```python
from build123d import *

# Parameters (mm, degrees)
F0_R     = 11
F1_DEPTH = 14.1
F2_R     = 11.385
F3_DEPTH = 28.4
F5_DEPTH = 17.5
F7_R     = 0.4828427125


# Not quite as in the source:
# - a fillet or chamfer that OpenCascade refuses, or shapes differently, is made with other operations: its cross-section is extruded or revolved along the edge and cut away or added


with BuildPart() as f1:
    # F0 (on Top) → F1 (new body)
    with BuildSketch(Plane.XY):
        with Locations((0, -12.3603016903)):
            Circle(F0_R)
    extrude(amount=F1_DEPTH)

    # F2 (on Front) → F3 (cut)
    with BuildSketch(Plane.XZ):
        with Locations((0, 18.905)):
            Circle(F2_R)
    extrude(amount=F3_DEPTH, mode=Mode.SUBTRACT)

    # F4 (on face) → F5 (join)
    with BuildSketch(Plane(origin=(0, 0, 0), x_dir=(1, 0, 0), z_dir=(0, 0, -1))):
        with BuildLine():
            ThreePointArc((0, 15.5053016903), (-3.145, 12.3603016903), (0, 9.2153016903))
            Line((0, 9.2153016903), (0, 15.5053016903))
        make_face()
        with BuildLine():
            Line((0, 15.5053016903), (0, 9.2153016903))
            ThreePointArc((0, 9.2153016903), (2.2238508268, 10.1364508634), (3.145, 12.3603016903))
            ThreePointArc((3.145, 12.3603016903), (2.2238508268, 14.5841525171), (0, 15.5053016903))
        make_face()
    extrude(amount=-F5_DEPTH)

    # F6: chamfer of 1 on 1 edges, made by hand

    # F6_s1 → F6_t2 (revolve, cut)
    with BuildSketch(Plane.YZ):
        Polygon((-9.2153016903, 16.5), (-10.2153016903, 17.5), (-9.2153016903, 17.5), align=None)
    revolve(axis=Axis((0, -12.3603016903, 17.5), (0, 0, -1)), mode=Mode.SUBTRACT)

    # F7
    f7_edges = [f1.edges().sort_by_distance(p)[0] for p in [
        (-11, -12.360302, 0),
    ]]
    fillet(f7_edges, radius=F7_R)

    # F8: chamfer of 0.4 on 1 edges, made by hand

    # F8_s1 → F8_t2 (revolve, cut)
    with BuildSketch(Plane.YZ):
        Polygon((-9.2153016903, 16.1), (-9.4981444028, 16.7828427125), (-9.2153016903, 16.5), align=None)
    revolve(axis=Axis((0, -12.3603016903, 16.5), (0, 0, -1)), mode=Mode.SUBTRACT)


solid = f1.part
```
Verification items for the finished model (mm, model axes). Round coordinates to 2 decimals unless told otherwise and drop trailing zeros. Write each loop counter-clockwise with the first axis right and the second up, starting at its lowest first coordinate (ties: lowest second). Pieces come first, ordered by that corner, then holes. Notation, with made-up numbers: (47, 59) -> (68, 59) arc R24 ccw to (68, 86) -> close; hole circle Ø1 at (-23.75, -23.75). An arc over 180 degrees is marked (long way). Write each question's results on one line, items separated by ' | '. Start each with the question number.
1. Material ranges on probe 1 along X at (y, z) = (-10, 13.5); probe 2 along X at (y, z) = (-19, 9.25); probe 3 along Y at (x, z) = (7.5, 8), recorded low to high. Write a range as from..to.
2. Cross-section at B-B (z = 5.25). Enter the section's corners in (x, y).
3. Draft check along X on faces 1 (the cylindrical face through (-3.016, -9.762, 7.927)), 2 (the flat face through (0, -12, 17.5)), 3 (the cylindrical face through (10.492, -9.056, 5.683)). Enter one of: +X half, -X half, draft (parallel to the pull), parting line (faces both ways), or undercut.
4. Depth check by flat-ended pin: P1, Ø1, axis at y = -21, z = 3, coming from the +X side; P2, Ø5, axis at x = -5.5, y = -13, coming from the +Z side; P3, Ø1, axis at x = 2.5, z = 8.5, coming from the +Y side. Enter the tip coordinate at first touch or a pass-through.
5. Cross-section at A-A (z = 10.25). Enter the section's corners in (x, y) (3 decimals).
Solutions:
1) probe 1: x = -10.74..-10.02, -2.08..2.08, 10.02..10.74 | probe 2: x = -8.77..-6.03, 6.03..8.77 | probe 3: y = -20.41..-4.31
2) outline: circle Ø22 at (0, -12.36)
3) face 1: undercut | face 2: draft | face 3: parting line
4) P1: stops at x = 7.4 | P2: stops at z = 16.36 | P3: stops at y = -9.93
5) outline: (-7.397, -20.502) -> (-7.397, -4.218) arc R11 ccw to start; circle Ø6.29 at (0, -12.36); (7.397, -20.502) arc R11 ccw to (7.397, -4.218) -> close
